Verification items for the finished model (mm, model axes). Face numbers are marked on the shaded views. A direction names the side the tool comes from. Give positions to 0.01 mm unless a question says otherwise; leave off trailing zeros. Loops run counter-clockwise (first coordinate to the right, second up) from the corner with the lowest first, then second, coordinate; pieces in that order, holes last. Notation, with made-up numbers: (3, 86) -> (40, 86) arc R36 cw to (40, 124) -> close; hole circle Ø5 at (83.5, 62.5). An arc over 180 degrees is marked (long way). Answer in a Markdown table with one row per item. Add a question column.
Q1. Section check B-B on x = 9. Enter the section's corners in (y, z), and give its area (3 significant figures).
Q2. Section check D-D on x = 26. Enter the section's corners in (y, z).
Q3. Set-up check for the marked faces 5, 6, 7, 8 and 9: record each of +Z, -Z, +X, -X, +Y, -Y from which the full face is reachable in a straight line by a thin tool's end or side.
Q4. Material ranges on probe 1 along X at (y, z) = (4.05, -12.25); probe 2 along X at (y, z) = (3.2, -23); probe 3 along X at (y, z) = (0.95, -24.75), recorded low to high.
Q5. Section check A-A on z = -23. Enter the section's corners in (x, y), and give its area (3 significant figures).
Q6. Gauge pin test, flat end, axial feed: P1, Ø1.5, axis at x = 57.5, y = 2, coming from the -Z side. Record the tip position at first contact, or that the pin passes through.
Q7. Section check C-C on y = 2.25. Enter the section's corners in (x, z).
Q8. Release check for a two-part mould opening along Z. For the marked faces 1, 2, 3 and 4 record: pulls with the +Z half, pulls with the -Z half, needs draft (parallel to the pull), parting line crosses it, or undercut.
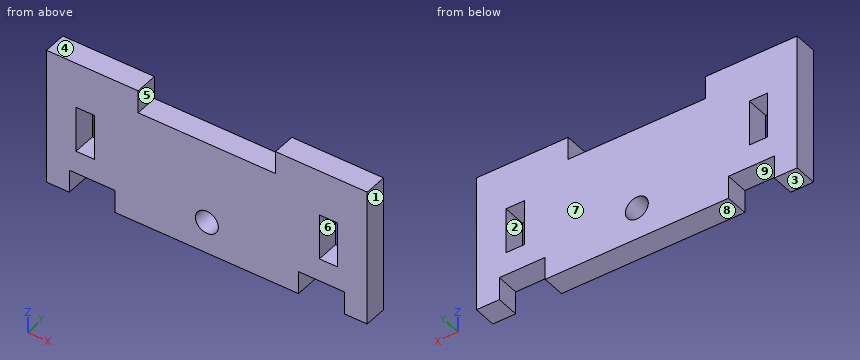
```python
from build123d import *

# Parameters (mm, degrees)
SKETCH_1_R      = 2.5
SKETCH_1_W      = 4
SKETCH_1_H      = 10
EXTRUDE_1_DEPTH = 5


with BuildPart() as part:
    # 草图1 → 凸台-拉伸1 (new body)
    with BuildSketch(Plane(origin=(0, 0, 0), x_dir=(1, 0, 0), z_dir=(0, 1, 0))):
        Polygon((0, 0), (20, 0), (20, 5), (50, 5), (50, 0), (70, 0), (70, 30), (65, 30), (65, 25), (55, 25), (55, 30), (15, 30), (15, 25), (5, 25), (5, 30), (0, 30), align=None)
        with Locations(Location((35, 23, 0), (0, 0, 270))):
            Circle(SKETCH_1_R, mode=Mode.SUBTRACT)
        with Locations((61.55, 15)):
            Rectangle(SKETCH_1_W, SKETCH_1_H, mode=Mode.SUBTRACT)
        with Locations((8.45, 15)):
            Rectangle(SKETCH_1_W, SKETCH_1_H, mode=Mode.SUBTRACT)
    extrude(amount=EXTRUDE_1_DEPTH)


solid = part.part
```
Taken from the geometry:
| question | item | result |
|---|---|---|
| 1 | outline | (0, -25) -> (5, -25) -> (5, -20) -> (0, -20) -> close; (0, -10) -> (5, -10) -> (5, 0) -> (0, 0) -> close |
| 1 | area | 75.0 mm² |
| 2 | outline | (0, -30) -> (5, -30) -> (5, -5) -> (0, -5) -> close |
| 3 | face 5 | +Z, +Y, -Y |
| 3 | face 6 | +Y, -Y |
| 3 | face 7 | +Z, -Z, +X, -X, +Y |
| 3 | face 8 | -Z, +X, -X, +Y, -Y |
| 3 | face 9 | -Z, +Y, -Y |
| 4 | probe 1 | x = 0 to 6.45, 10.45 to 59.55, 63.55 to 70 |
| 4 | probe 2 | x = 0 to 32.5, 37.5 to 70 |
| 4 | probe 3 | x = 0 to 33.21, 36.79 to 70 |
| 5 | outline | (0, 0) -> (32.5, 0) -> (32.5, 5) -> (0, 5) -> close; (37.5, 0) -> (70, 0) -> (70, 5) -> (37.5, 5) -> close |
| 5 | area | 325 mm² |
| 6 | P1 | stops at z = -25 |
| 7 | outline | (0, -30) -> (5, -30) -> (5, -25) -> (15, -25) -> (15, -30) -> (55, -30) -> (55, -25) -> (65, -25) -> (65, -30) -> (70, -30) -> (70, 0) -> (50, 0) -> (50, -5) -> (20, -5) -> (20, 0) -> (0, 0) -> close; hole (6.45, -20) -> (10.45, -20) -> (10.45, -10) -> (6.45, -10) -> close; hole circle Ø5 at (35, -23); hole (59.55, -20) -> (63.55, -20) -> (63.55, -10) -> (59.55, -10) -> close |
| 8 | face 1 | needs draft |
| 8 | face 2 | undercut |
| 8 | face 3 | pulls with the -Z half |
| 8 | face 4 | pulls with the +Z half |
